Input: part model. Units: mm. Frame: model coordinates. A direction names the side the tool comes from. Give positions to 0.01 mm unless a question says otherwise; leave off trailing zeros. Order: outer loops, then holes, each group sorted by start corner. A loop starts at its lowest first (then second) coordinate and runs counter-clockwise, first axis right, second up.
```python
from build123d import *

# Parameters (mm, degrees)
SKETCH_1_W                   = 320
SKETCH_1_H                   = 50
EXTRUDE_1_DEPTH              = 14
HOLE_WIZARD_M6_1_D           = 6.6
HOLE_WIZARD_M6_1_CBORE_D     = 11
HOLE_WIZARD_M6_1_CBORE_DEPTH = 6.4
SKETCH_5_R                   = 6
CUT_EXTRUDE_1_DEPTH          = 3
SKETCH_6_W                   = 8
SKETCH_6_H                   = 50
CUT_EXTRUDE_2_DEPTH          = 1
HOLE_WIZARD_M5_1_D           = 5.5
HOLE_WIZARD_M5_1_CBORE_D     = 10
HOLE_WIZARD_M5_1_CBORE_DEPTH = 5.4
SKETCH_9_W                   = 30
SKETCH_9_H                   = 14
CUT_EXTRUDE_3_DEPTH          = 15
SKETCH_10_W                  = 120
SKETCH_10_H                  = 100
SKETCH_10_R                  = 39
EXTRUDE_2_DEPTH              = 14
SKETCH_15_R                  = 39
EXTRUDE_3_DEPTH              = 14
CUT_EXTRUDE_4_DEPTH          = 31.5
SKETCH_17_W                  = 120
SKETCH_17_H                  = 14
EXTRUDE_4_DEPTH              = 14.2
SKETCH_18_W                  = 120
SKETCH_18_H                  = 14
EXTRUDE_5_DEPTH              = 10
HOLE_WIZARD_M5_1_2_D         = 4.2
HOLE_WIZARD_M5_1_2_DEPTH     = 12.4
HOLE_WIZARD_M5_1_2_TIP       = 1.2618073
SKETCH_21_W                  = 21
SKETCH_21_H                  = 124.2
CUT_EXTRUDE_5_DEPTH          = 1
HOLE_WIZARD_M5_2_D           = 4.2
HOLE_WIZARD_M5_2_DEPTH       = 12.4
HOLE_WIZARD_M5_2_TIP         = 1.2618073


with BuildPart() as part:
    # 草图1 → 凸台-拉伸1 (new body)
    with BuildSketch(Plane.XY):
        with Locations((160, 25)):
            Rectangle(SKETCH_1_W, SKETCH_1_H)
    extrude(amount=EXTRUDE_1_DEPTH)

    # M6 六角凹头螺钉的柱形沉头孔1 (through all)
    with Locations(Plane.XY.offset(14)):
        with Locations((283, 25), (37, 25)):
            CounterBoreHole(HOLE_WIZARD_M6_1_D / 2, HOLE_WIZARD_M6_1_CBORE_D / 2, HOLE_WIZARD_M6_1_CBORE_DEPTH)

    # 草图5 → 切除-拉伸1 (cut)
    with BuildSketch(Plane(origin=(0, 0, 0), x_dir=(-1, 0, 0), z_dir=(0, 0, -1))):
        with Locations((-283, 25)):
            Circle(SKETCH_5_R)
        with Locations((-37, 25)):
            Circle(SKETCH_5_R)
    extrude(amount=-CUT_EXTRUDE_1_DEPTH, mode=Mode.SUBTRACT)

    # 草图6 → 切除-拉伸2 (cut)
    with BuildSketch(Plane(origin=(0, 0, 0), x_dir=(-1, 0, 0), z_dir=(0, 0, -1))):
        with Locations((-9, 25)):
            Rectangle(SKETCH_6_W, SKETCH_6_H)
        with Locations((-311, 25)):
            Rectangle(SKETCH_6_W, SKETCH_6_H)
    extrude(amount=-CUT_EXTRUDE_2_DEPTH, mode=Mode.SUBTRACT)

    # Hole Wizard M5 _1 (through all)
    with Locations(Plane.XY.offset(14)):
        with Locations((311, 10), (311, 40), (9, 40), (9, 10)):
            CounterBoreHole(HOLE_WIZARD_M5_1_D / 2, HOLE_WIZARD_M5_1_CBORE_D / 2, HOLE_WIZARD_M5_1_CBORE_DEPTH)

    # 草图9 → 切除-拉伸3 (cut)
    with BuildSketch(Plane.XZ):
        with Locations((160, 7)):
            Rectangle(SKETCH_9_W, SKETCH_9_H)
    extrude(amount=-CUT_EXTRUDE_3_DEPTH, mode=Mode.SUBTRACT)

    # 草图10 → 凸台-拉伸2 (add)
    with BuildSketch(Plane.XY.offset(14)):
        with Locations((160, 25)):
            Rectangle(SKETCH_10_W, SKETCH_10_H)
        with Locations((160, 25)):
            Circle(SKETCH_10_R, mode=Mode.SUBTRACT)
    extrude(amount=-EXTRUDE_2_DEPTH)

    # 草图15 → 凸台-拉伸3 (add)
    with BuildSketch(Plane.XY.offset(14)):
        with Locations((160, 25)):
            Circle(SKETCH_15_R)
    extrude(amount=-EXTRUDE_3_DEPTH)

    # 草图16 → 切除-拉伸4 (cut)
    with BuildSketch(Plane.XY.offset(14)):
        with BuildLine():
            Line((185, 10), (185, 40))
            ThreePointArc((185, 40), (160, 65), (135, 40))
            Line((135, 40), (135, 10))
            ThreePointArc((135, 10), (160, -15), (185, 10))
        make_face()
    extrude(amount=-CUT_EXTRUDE_4_DEPTH, mode=Mode.SUBTRACT)

    # 草图17 → 凸台-拉伸4 (add)
    with BuildSketch(Plane.XZ.offset(25)):
        with Locations((160, 7)):
            Rectangle(SKETCH_17_W, SKETCH_17_H)
    extrude(amount=EXTRUDE_4_DEPTH)

    # 草图18 → 凸台-拉伸5 (add)
    with BuildSketch(Plane(origin=(0, 75, 0), x_dir=(1, 0, 0), z_dir=(0, 1, 0))):
        with Locations((160, -7)):
            Rectangle(SKETCH_18_W, SKETCH_18_H)
    extrude(amount=EXTRUDE_5_DEPTH)

    # Hole Wizard M5 _1 2
    with Locations(Plane.XY.offset(14)):
        with Locations((121, -3), (121, -23)):
            Hole(HOLE_WIZARD_M5_1_2_D / 2, depth=HOLE_WIZARD_M5_1_2_DEPTH)
            with Locations((0, 0, -(HOLE_WIZARD_M5_1_2_DEPTH + HOLE_WIZARD_M5_1_2_TIP / 2))):  # 118° drill point
                Cone(0, HOLE_WIZARD_M5_1_2_D / 2, HOLE_WIZARD_M5_1_2_TIP, mode=Mode.SUBTRACT)

    # 草图21 → 切除-拉伸5 (cut)
    with BuildSketch(Plane.XY.offset(14)):
        with Locations((124, 22.9)):
            Rectangle(SKETCH_21_W, SKETCH_21_H)
    extrude(amount=-CUT_EXTRUDE_5_DEPTH, mode=Mode.SUBTRACT)

    # M5 螺纹孔2
    with Locations(Plane(origin=(0, -39.2, 0), x_dir=(-1, 0, 0), z_dir=(0, -1, 0))):
        with Locations((-160, -7), (-110, -7), (-210, -7)):
            Hole(HOLE_WIZARD_M5_2_D / 2, depth=HOLE_WIZARD_M5_2_DEPTH)
            with Locations((0, 0, -(HOLE_WIZARD_M5_2_DEPTH + HOLE_WIZARD_M5_2_TIP / 2))):  # 118° drill point
                Cone(0, HOLE_WIZARD_M5_2_D / 2, HOLE_WIZARD_M5_2_TIP, mode=Mode.SUBTRACT)


solid = part.part
```
1) Cut plane B-B (y = 70.5). Return the cut outline in (x, z).
2) First-contact query: P1, Ø2, axis at y = -11.5, z = 4, coming from the +X side; P2, Ø4, axis at x = 284, z = 6.5, coming from the +Y side; P3, Ø3.5, axis at x = 121, y = -23, coming from the +Z side. Flat tips, straight axial feed; report the tip coordinate or a pass-through.
3) Pull-direction query (X, two-part tool) for faces 1 (the face through (49, 0, 7)), 2 (the face through (320, 25, 7)), 3 (the face through (287, 25, 7.6)), 4 (the face through (185, 25, 7)); classes: pulls with the +X half, pulls with the -X half, needs draft (parallel to the pull), parting line crosses it, or undercut.
4) Reachability of faces 5 (the face through (41, 25, 7.6)), 6 (the face through (9, 25, 1)), 7 (the face through (226, 22, 14)), 8 (the face through (280, 22, 3)), 9 (the face through (124, 24, 13)) from +Z, -Z, +X, -X, +Y, -Y: full face, straight path, thin tool, end or side. Return the list, or none.
5) Cut plane A-A (x = 175). Return the cut outline in (y, z).
6) Cut plane D-D (x = 273.5). Return the cut outline in (y, z).
7) Cut plane C-C (x = 9). Return the cut outline in (y, z), then the cut area to 3 significant figures.
8) Line query: probe 1 along Y at (x, z) = (121, 11.75); probe 2 along Y at (x, z) = (9, 10.8); probe 3 along Y at (x, z) = (37, 1.8). Output: solid intervals per line, ascending.
Geometry says:
1. outline: (100, 0) - (220, 0) - (220, 14) - (134.5, 14) - (134.5, 13) - (113.5, 13) - (113.5, 14) - (100, 14) - close
2. P1: stops at x = 220
2. P2: stops at y = 50
2. P3: stops at z = 1.39
3. face 1: needs draft
3. face 2: pulls with the +X half
3. face 3: undercut
3. face 4: undercut
4. face 5: +Z
4. face 6: -Z, +Y, -Y
4. face 7: +Z, +X, -X, +Y, -Y
4. face 8: -Z
4. face 9: +Z, +Y, -Y
5. outline: (-39.2, 0) - (-10, 0) - (-10, 14) - (-39.2, 14) - close; (60, 0) - (85, 0) - (85, 14) - (60, 14) - close
6. outline: (0, 0) - (50, 0) - (50, 14) - (0, 14) - close
7. outline: (0, 1) - (7.25, 1) - (7.25, 8.6) - (5, 8.6) - (5, 14) - (0, 14) - close; (12.75, 1) - (37.25, 1) - (37.25, 8.6) - (35, 8.6) - (35, 14) - (15, 14) - (15, 8.6) - (12.75, 8.6) - close; (42.75, 1) - (50, 1) - (50, 14) - (45, 14) - (45, 8.6) - (42.75, 8.6) - close
7. area: 458 mm2
8. probe 1: y = -39.2 to -25.1, -20.9 to -5.1, -0.9 to 85
8. probe 2: y = 0 to 5, 15 to 35, 45 to 50
8. probe 3: y = 0 to 19, 31 to 50
